For this review, take the finished solid that the model builds, in its own axes (mm). A direction names the side the tool comes from. Give positions to 0.01 mm unless a question says otherwise; leave off trailing zeros. Write each loop counter-clockwise with the first axis right and the second up, starting at its lowest first coordinate (ties: lowest second). Pieces come first, ordered by that corner, then holes. Notation, with made-up numbers: M 84.25,61.25 L 100.25,61.25 A18 cw 100.25,79.25 Z; hole C 8,86 d11. An arc over 180 degrees is marked long. Write item = value, one per line.
```python
from build123d import *

# Parameters (mm, degrees)
SKETCH_1_R          = 16
EXTRUDE_1_DEPTH     = 2
SKETCH_2_R          = 25.05
EXTRUDE_2_DEPTH     = 15
SKETCH_4_R          = 2
CUT_EXTRUDE_1_DEPTH = 10
SKETCH_6_W          = 60
SKETCH_6_H          = 1.5
CUT_EXTRUDE_2_DEPTH = 1.5
SKETCH_8_R          = 10
CUT_EXTRUDE_3_DEPTH = 2


with BuildPart() as part:
    # 草图1 → 凸台-拉伸1 (new body)
    with BuildSketch(Plane(origin=(0, 0, 0), x_dir=(1, 0, 0), z_dir=(0, 1, 0))):
        with Locations(Location((0, 0, 0), (0, 0, 270))):
            Circle(SKETCH_1_R)
    extrude(amount=-EXTRUDE_1_DEPTH)

    # 草图2 → 凸台-拉伸2 (add)
    with BuildSketch(Plane.XZ.offset(2)):
        with Locations(Location((0, 0, 0), (0, 0, 270))):
            Circle(SKETCH_2_R)
    extrude(amount=EXTRUDE_2_DEPTH)

    # 草图4 → 切除-拉伸1 (cut)
    with BuildSketch(Plane.XZ.offset(17)):
        with Locations(Location((0, 0, 0), (0, 0, 270))):
            Circle(SKETCH_4_R)
    extrude(amount=-CUT_EXTRUDE_1_DEPTH, mode=Mode.SUBTRACT)

    # 草图6 → 切除-拉伸2 (cut)
    with BuildSketch(Plane(origin=(0, -2, 0), x_dir=(1, 0, 0), z_dir=(0, 1, 0))):
        Rectangle(SKETCH_6_W, SKETCH_6_H)
    extrude(amount=CUT_EXTRUDE_2_DEPTH, mode=Mode.SUBTRACT)

    # 草图8 → 切除-拉伸3 (cut)
    with BuildSketch(Plane(origin=(0, 0, 0), x_dir=(1, 0, 0), z_dir=(0, 1, 0))):
        with Locations(Location((0, 0, 0), (0, 0, 270))):
            Circle(SKETCH_8_R)
    extrude(amount=-CUT_EXTRUDE_3_DEPTH, mode=Mode.SUBTRACT)


solid = part.part
```
1. Insertion check: P1, Ø1.6, axis at x = -13.5, y = -1.5, coming from the -Z side; P2, Ø1.6, axis at x = 12, y = -1.5, coming from the +Z side; P3, Ø1.5, axis at x = -17.5, y = -9.5, coming from the +Z side. Each pin has a flat end and moves straight along its axis. Give the tip position at first contact, or say it passes through.
Responses:
P1 = -21.49
P2 = 22.32
P3 = 18.63
2. The part is to be moulded in two halves that separate along Y. For faces 1 (the face through (13, -1, -0.75)), 2 (the face through (0, -7, 0)), 3 (the face through (-2, -12, 0)), say which applies: +Y half, -Y half, draft (parallel to the pull), parting line (faces both ways), or undercut.
Responses:
face_1 = undercut
face_2 = -Y half
face_3 = draft
3. For line 1 along X through (y, z) = (-13.5, 0); line 2 along Z through (x, y) = (0, -1.4); line 3 along Y through (x, z) = (22.5, 10), list the stretches that pass through material, from the lowest coordinate up. Write a range as from..to.
Responses:
line_1 = -25.05..-2, 2..25.05
line_2 = -16..-10, 10..16
line_3 = -17..-2
4. We need section C-C, the plane y = -8.5. Write out the cut boundary in (x, z).
Responses:
outline = C 0,0 d50.1; hole C 0,0 d4
5. We need section A-A, the plane z = 0. Write out the cut boundary in (x, y), then the cut area to 4 significant figures.
Responses:
outline = M -25.05,-17 L -2,-17 L -2,-7 L 2,-7 L 2,-17 L 25.05,-17 L 25.05,-2 L -25.05,-2 Z; M -16,-0.5 L -10,-0.5 L -10,0 L -16,0 Z; M 10,-0.5 L 16,-0.5 L 16,0 L 10,0 Z
area = 717.5 mm2
6. We need section D-D, the plane z = 14. Write out the cut boundary in (x, y), then the cut area to 3 significant figures.
Responses:
outline = M -20.77,-17 L 20.77,-17 L 20.77,-2 L 7.75,-2 L 7.75,0 L -7.75,0 L -7.75,-2 L -20.77,-2 Z
area = 654 mm2
7. Machinability: for faces 4 (the face through (13, -0.5, 0)), 5 (the face through (-9.76, -0.99, -2.17)), 6 (the face through (-10.4, 0, -0.2)), which of the approach directions +Z, -Z, +X, -X, +Y, -Y give a long, thin tool a straight path to every point of the face, cutting with its end or side? Answer none if there is none.
Responses:
face_4 = +X, -X
face_5 = +Y
face_6 = +Z, -Z, +X, -X, +Y
8. We need section B-B, the plane x = 0. Write out the cut boundary in (y, z), then the cut area to 4 significant figures.
Responses:
outline = M -17,-25.05 L -2,-25.05 L -2,-16 L 0,-16 L 0,-10 L -2,-10 L -2,10 L 0,10 L 0,16 L -2,16 L -2,25.05 L -17,25.05 L -17,2 L -7,2 L -7,-2 L -17,-2 Z
area = 735.5 mm2
